Can you work these out from the model? Positions are in its coordinate system, mm. Face numbers are marked on the shaded views. A direction names the side the tool comes from. Give positions to 0.01 mm unless a question says otherwise; leave off trailing zeros. Loops run counter-clockwise (first coordinate to the right, second up) from the corner with the lowest first, then second, coordinate; pieces in that order, holes last. Notation, with made-up numbers: (84.5, 41) - (121.5, 41) arc R22 ccw to (121.5, 47) - close; hole circle Ø3 at (-33.75, -29). An arc over 180 degrees is marked (long way). Answer as a JSON object with one key per item and string values.
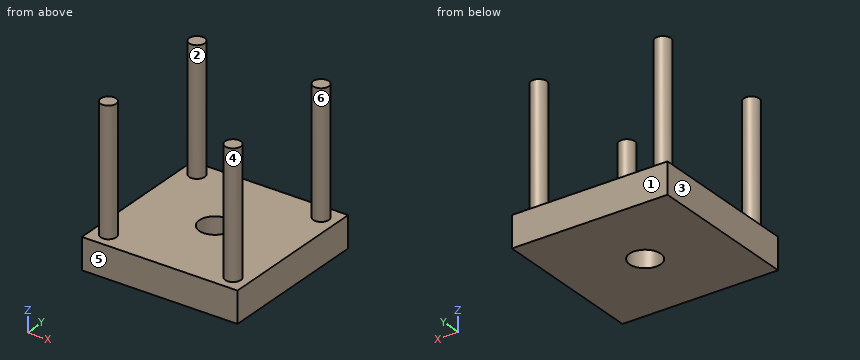
```python
from build123d import *

# Parameters (mm, degrees)
F0_R     = 0.5
F0_R_2   = 1
F1_DEPTH = 2
F2_DEPTH = 10


with BuildPart() as f1:
    # F0 (on Top) → F1 (new body)
    with BuildSketch(Plane.XY):
        Polygon((5.029937, -5.029937), (5.029937, 4.970063), (-4.970063, 4.970063), (-4.970063, -0.907308), (-4.970063, -5.029937), align=None)
        with Locations((-3.970063, -4.029937)):
            Circle(F0_R, mode=Mode.SUBTRACT)
        with Locations((4.016325, -4.009387)):
            Circle(F0_R, mode=Mode.SUBTRACT)
        Circle(F0_R_2, mode=Mode.SUBTRACT)
        with Locations((-3.970063, 3.970063)):
            Circle(F0_R, mode=Mode.SUBTRACT)
        with Locations((4.016325, 3.949514)):
            Circle(F0_R, mode=Mode.SUBTRACT)
    extrude(amount=F1_DEPTH)

    # F0 (on Top) → F2 (join)
    with BuildSketch(Plane.XY):
        with Locations((-3.970063, 3.970063)):
            Circle(F0_R)
        with Locations((4.016325, 3.949514)):
            Circle(F0_R)
        with Locations((4.016325, -4.009387)):
            Circle(F0_R)
        with Locations((-3.970063, -4.029937)):
            Circle(F0_R)
    extrude(amount=F2_DEPTH)


solid = f1.part
```
1) I'm going to push flat-ended pins straight in: P1, Ø2, axis at x = -1, y = 0, coming from the -Z side; P2, Ø2, axis at x = -4, z = 4.5, coming from the -Y side; P3, Ø3, axis at y = 0.5, z = 8.5, coming from the -X side. Where does each tip first touch, or does it pass through?
Check sheet entries:
{"P1": "z = 0", "P2": "y = -4.53", "P3": "through"}
2) Imagine slicing it at D-D on y = -2.5. Write out the boundary of the cut face in (x, z), and give its area (3 significant figures).
Check sheet entries:
{"outline": "(-4.97, 0) - (5.03, 0) - (5.03, 2) - (-4.97, 2) - close", "area": "20.0 mm2"}
3) Imagine slicing it at B-B on x = 0. Write out the boundary of the cut face in (y, z).
Check sheet entries:
{"outline": "(-5.03, 0) - (-1, 0) - (-1, 2) - (-5.03, 2) - close; (1, 0) - (4.97, 0) - (4.97, 2) - (1, 2) - close"}
4) I need wall thicknesses on L1, parallel to Y at x = 0, z = 1.4; L2, parallel to Y at x = -4, z = 4; L3, parallel to Z at x = -3.75, y = -2.5. Which ranges of each line are inside material? Lowest first, please.
Check sheet entries:
{"L1": "-5.03 to -1, 1 to 4.97", "L2": "-4.53 to -3.53, 3.47 to 4.47", "L3": "0 to 2"}
5) Imagine slicing it at C-C on z = 1.75. Write out the boundary of the cut face in (x, y).
Check sheet entries:
{"outline": "(-4.97, -5.03) - (5.03, -5.03) - (5.03, 4.97) - (-4.97, 4.97) - close; hole circle Ø2 at (0, 0)"}
6) If we mould it in two halves opening along Y, with no side actions, what happens to the marked faces 3, 4, 5 and 6? For each: released by +Y, released by -Y, zero draft, split by the parting line, or undercut.
Check sheet entries:
{"face 3": "zero draft", "face 4": "undercut", "face 5": "released by -Y", "face 6": "undercut"}
7) Imagine slicing it at A-A on y = 0. Write out the boundary of the cut face in (x, z), and give its area (3 significant figures).
Check sheet entries:
{"outline": "(-4.97, 0) - (-1, 0) - (-1, 2) - (-4.97, 2) - close; (1, 0) - (5.03, 0) - (5.03, 2) - (1, 2) - close", "area": "16.0 mm2"}
8) Which directions (+Z, -Z, +X, -X, +Y, -Y) give clear straight access to the entire face, cutting with the end or side of a thin tool? Please do the marked faces 1 and 2.
Check sheet entries:
{"face 1": "+Z, -Z, +X, -X, +Y", "face 2": "+Z"}
